from build123d import *

# Parameters (mm, degrees)
PAD007_DEPTH    = 1.5
PAD008_DEPTH    = 0.5
SKETCH012_W     = 5
SKETCH012_H     = 2.5
SKETCH012_W_2   = 7.5
PAD009_DEPTH    = 0.8
SKETCH013_W     = 7.5
SKETCH013_H     = 3
PAD010_DEPTH    = 0.5
POCKET003_DEPTH = 0.5
POCKET004_DEPTH = 2
SKETCH021_W     = 5
SKETCH021_H     = 8
PAD013_DEPTH    = 3.2
SKETCH024_R     = 2.6
POCKET007_DEPTH = 5.201


with BuildPart() as part:
    # Sketch010 → Pad007 (new body)
    with BuildSketch(Plane.XY.offset(-19)):
        with BuildLine():
            Line((-29.25, 12.75), (29.25, 12.75))
            ThreePointArc((33, 9), (31.9016504294, 11.6516504294), (29.25, 12.75))
            Line((33, 9), (33, -9))
            ThreePointArc((29.25, -12.75), (31.9016504295, -11.6516504294), (33, -9))
            Line((29.25, -12.75), (-29.25, -12.75))
            ThreePointArc((-33, -9), (-31.9016504294, -11.6516504295), (-29.25, -12.75))
            Line((-33, -9), (-33, 9))
            ThreePointArc((-29.25, 12.75), (-31.9016504294, 11.6516504294), (-33, 9))
        make_face()
    extrude(amount=PAD007_DEPTH)

    # Sketch011 → Pad008 (new body)
    with BuildSketch(Plane.XY.offset(-17.5)):
        with BuildLine():
            Line((-29.05, 11.05), (29.05, 11.05))
            ThreePointArc((31.3, 8.8), (30.6409902577, 10.3909902577), (29.05, 11.05))
            Line((31.3, 8.8), (31.3, -8.8))
            ThreePointArc((29.05, -11.05), (30.6409902577, -10.3909902577), (31.3, -8.8))
            Line((29.05, -11.05), (-29.05, -11.05))
            ThreePointArc((-31.3, -8.8), (-30.6409902577, -10.3909902577), (-29.05, -11.05))
            Line((-31.3, -8.8), (-31.3, 8.8))
            ThreePointArc((-29.05, 11.05), (-30.6409902577, 10.3909902577), (-31.3, 8.8))
        make_face()
    extrude(amount=PAD008_DEPTH)

    # Sketch012 → Pad009 (new body)
    with BuildSketch(Plane.XY.offset(-17)):
        with Locations((-10.5, 10.3)):
            Rectangle(SKETCH012_W, SKETCH012_H)
        with Locations((10.5, 10.3)):
            Rectangle(SKETCH012_W, SKETCH012_H)
        with Locations((0, -9.75)):
            Rectangle(SKETCH012_W_2, SKETCH012_H)
    extrude(amount=PAD009_DEPTH)

    # Sketch013 → Pad010 (new body)
    with BuildSketch(Plane.XY.offset(-16.2)):
        with Locations((0, -10)):
            Rectangle(SKETCH013_W, SKETCH013_H)
    extrude(amount=PAD010_DEPTH)

    # Sketch016 → Pocket003 (cut)
    with BuildSketch(Plane.XY.offset(-17)):
        with BuildLine():
            ThreePointArc((28.00000543, -6.5), (26.2322368866, -7.2322292075), (25.5, -8.99999457))
            ThreePointArc((23.4499998257, -11.05), (24.8995699389, -10.4495662225), (25.5, -8.99999457))
            Line((23.4499998257, -11.25), (23.4499998257, -11.05))
            Line((31.5, -11.25), (23.4499998257, -11.25))
            Line((31.5, -3.1999998258), (31.5, -11.25))
            Line((31.3, -3.1999998258), (31.5, -3.1999998258))
            ThreePointArc((28.00000543, -6.5), (30.3334594583, -5.5334554955), (31.3, -3.1999998258))
        make_face()
        with BuildLine():
            Line((-23.4499998257, 11.05), (-23.4499998257, 11.25))
            Line((-23.4499998257, 11.25), (-31.5, 11.25))
            Line((-31.5, 11.25), (-31.5, 3.1999998257))
            Line((-31.5, 3.1999998257), (-31.3, 3.1999998257))
            ThreePointArc((-27.9999999386, 6.5), (-30.3334523833, 5.5334523035), (-31.3, 3.1999998257))
            ThreePointArc((-27.9999999386, 6.5), (-26.2322330036, 7.2322330904), (-25.5, 9.0000000614))
            ThreePointArc((-23.4499998257, 11.05), (-24.8995688016, 10.4495689682), (-25.5, 9.0000000614))
        make_face()
    extrude(amount=-POCKET003_DEPTH, mode=Mode.SUBTRACT)

    # Sketch017 → Pocket004 (cut)
    with BuildSketch(Plane.XY.offset(-17)):
        with BuildLine():
            ThreePointArc((-24, -6.1), (-25.2, -7.3), (-24, -8.5))
            Line((-24, -8.5), (24, -8.5))
            ThreePointArc((24, -8.5), (25.2, -7.3), (24, -6.1))
            Line((-24, -6.1), (24, -6.1))
        make_face()
    extrude(amount=-POCKET004_DEPTH, mode=Mode.SUBTRACT)

    # Sketch021 → Pad013 (new body)
    with BuildSketch(Plane.XY.offset(-17)):
        with Locations((28.8, 0)):
            Rectangle(SKETCH021_W, SKETCH021_H)
    extrude(amount=PAD013_DEPTH)

    # Sketch024 → Pocket007 (cut, through all)
    with BuildSketch(Plane(origin=(0, 0, -19), x_dir=(1, 0, 0), z_dir=(0, 0, -1))):
        with Locations((-19.9, -9.1)):
            Circle(SKETCH024_R)
    extrude(amount=-POCKET007_DEPTH, mode=Mode.SUBTRACT)


solid = part.part
Can you work these out from the model? Positions are in its coordinate system, mm. A direction names the side the tool comes from. Give positions to 0.01 mm unless a question says otherwise; leave off trailing zeros. Loops run counter-clockwise (first coordinate to the right, second up) from the corner with the lowest first, then second, coordinate; pieces in that order, holes last. Notation, with made-up numbers: (-9, -4.75) - (9, -4.75) arc R24 ccw to (9, 30.25) - close; hole circle Ø2 at (-26.75, 84). An arc over 180 degrees is marked (long way). Answer as a JSON object with one key per item and string values.
Q1. If we mould it in two halves opening along Y, with no side actions, what happens to faces 6 (the flat face through (0, 0, -19)), 7 (the flat face through (0, 12.75, -18)), 8 (the flat face through (0, -8.5, -18))? For each: pulls with the +Y half, pulls with the -Y half, needs draft (parallel to the pull), parting line crosses it, or undercut.
Geometry says:
{"face 6": "needs draft", "face 7": "pulls with the +Y half", "face 8": "undercut"}
Q2. Imagine slicing it at B-B on y = 1.75. Write out the boundary of the cut face in (x, z).
Geometry says:
{"outline": "(-33, -19) - (33, -19) - (33, -17.5) - (31.3, -17.5) - (31.3, -13.8) - (26.3, -13.8) - (26.3, -17) - (-31.3, -17) - (-31.3, -17.5) - (-33, -17.5) - close"}
Q3. Imagine slicing it at D-D on y = -7.3. Write out the boundary of the cut face in (x, z).
Geometry says:
{"outline": "(-33, -19) - (-25.2, -19) - (-25.2, -17) - (-31.3, -17) - (-31.3, -17.5) - (-33, -17.5) - close; (25.2, -19) - (33, -19) - (33, -17.5) - (26.17, -17.5) - (26.17, -17) - (25.2, -17) - close"}
Q4. Which directions (+Z, -Z, +X, -X, +Y, -Y) give clear straight access to the entire face, cutting with the end or side of a thin tool? Please do faces 1 (the flat face through (3.75, -10, -16)), 2 (the cylindrical face through (30.66, 10.37, -17.25)), 3 (the cylindrical face through (24.88, -10.47, -17.25)), 4 (the flat face through (0, -6.1, -18)), 5 (the cylindrical face through (-30.308, 5.559, -17.246)).
Geometry says:
{"face 1": "+Z, +X, +Y, -Y", "face 2": "+Z, +X, +Y", "face 3": "+Z, +X, -Y", "face 4": "+Z, -Z", "face 5": "+Z, -X, +Y"}
Q5. Imagine slicing it at A-A on x = 0.5. Write out the boundary of the cut face in (y, z), plus the area to 3 significant figures.
Geometry says:
{"outline": "(-12.75, -19) - (-8.5, -19) - (-8.5, -15.7) - (-11.5, -15.7) - (-11.5, -16.2) - (-11, -16.2) - (-11, -17) - (-11.05, -17) - (-11.05, -17.5) - (-12.75, -17.5) - close; (-6.1, -19) - (12.75, -19) - (12.75, -17.5) - (11.05, -17.5) - (11.05, -17) - (-6.1, -17) - close", "area": "48.0 mm²"}
Q6. Will these pins go through, and if not, where does the flat tip stop? P1, Ø3, axis at x = 11.5, y = 10.5, coming from the +Z side; P2, Ø0.9, axis at x = -10, z = -16.5, coming from the +Y side; P3, Ø7.5, axis at x = 1, y = 2.5, coming from the +Z side; P4, Ø2, axis at x = 23.5, z = -17, coming from the -Y side.
Geometry says:
{"P1": "z = -16.2", "P2": "y = 11.55", "P3": "z = -17", "P4": "y = -12.75"}
Q7. Imagine slicing it at C-C on x = -19.9. Write out the boundary of the cut face in (y, z), plus the area to 3 significant figures.
Geometry says:
{"outline": "(-12.75, -19) - (-8.5, -19) - (-8.5, -17) - (-11.05, -17) - (-11.05, -17.5) - (-12.75, -17.5) - close; (-6.1, -19) - (6.5, -19) - (6.5, -17) - (-6.1, -17) - close; (11.7, -19) - (12.75, -19) - (12.75, -17.5) - (11.7, -17.5) - close", "area": "34.4 mm²"}
Q8. If I drill on L1, parallel to Y at x = -19.9, z = -18.4; L2, parallel to X at y = 9.1, z = -17.75; L3, parallel to Y at x = -21, z = -18.75, over which ranges is the centre line in solid material (lowest first)?
Geometry says:
{"L1": "-12.75 to -8.5, -6.1 to 6.5, 11.7 to 12.75", "L2": "-33 to -22.5, -17.3 to 33", "L3": "-12.75 to -8.5, -6.1 to 6.74, 11.46 to 12.75"}
